Model file for the job. Use its own axes, mm. A direction names the side the tool comes from. Round coordinates to 2 decimals unless told otherwise and drop trailing zeros. Put each result on its own line as item: value. Start each with the question number.
Item 1: Pin check, flat tips, straight feed: pin 1 Ø8 at (x, y) = (124, 31.57) entering from -Z; pin 2 Ø7 at (x, y) = (124, 33.5) entering from -Z; pin 3 Ø6 at (x, y) = (136.5, 17) entering from -Z; pin 4 Ø4 at (y, z) = (27.5, 3.5) entering from -X. Stop position of each tip, or through.
Item 2: Mould opens along Y. For faces 1 (the face through (134.33, 18.47, 3.53)), 2 (the face through (146.229, 21, -4)), 3 (the face through (104.15, 5.837, -9.68)) say: pulls with the +Y half, pulls with the -Y half, needs draft (parallel to the pull), parting line crosses it, or undercut.
Item 3: Which spindle directions (+Z, -Z, +X, -X, +Y, -Y) get a long thin tool onto all of the face, cutting with end or side? Do faces 4 (the face through (128, 11, 1.27)), 5 (the face through (102.2, 21.2, -10.6)). Say none if no direction does.
Item 4: Probe probe 1 along Y at (x, z) = (116.5, -5.5); probe 2 along X at (y, z) = (17.5, -2); probe 3 along X at (y, z) = (19, -2.75). List the from-to ranges inside material, lowest first.
Item 5: Saw through at B-B on z = -2.75. State how many separate pieces and enclosed holes the cut face has, plus the area to 3 significant figures.
```python
from build123d import *

# Parameters (mm, degrees)
SKETCH1_W                   = 44.45
SKETCH1_H                   = 33.86758938
SKETCH1_W_2                 = 38.1
SKETCH1_H_2                 = 32.59758938
BOSS_EXTRUDE1_DEPTH         = 6.35
SKETCH2_W                   = 44.45
SKETCH2_H                   = 33.86758938
BOSS_EXTRUDE2_DEPTH         = 9.525
CUT_EXTRUDE1_DEPTH          = 151.402114191
SKETCH4_W                   = 3.175
SKETCH4_H                   = 33.86758938
BOSS_EXTRUDE3_DEPTH         = 4.7625
SHELL2_START                = 9.24120531
SHELL2_DEPTH                = 24.34258938
FILLET4_R                   = 4.7625
FILLET1_R                   = 4.7625
FILLET3_R                   = 6.35
FILLET2_R                   = 1.5875
F_10_CLEARANCE_HOLE1_D      = 5.6134
F_10_CLEARANCE_HOLE1_DEPTH  = 7.802129636
BOSS_EXTRUDE4_REACH         = 152.369
CUT_EXTRUDE2_START          = -4.7625
SKETCH9_R                   = 6.82625
CUT_EXTRUDE2_DEPTH          = 145.161286958
HOLE1_AT_2_COUNT            = 2
HOLE1_AT_2_PITCH            = 20.32
F_1_4_CLEARANCE_HOLE1_D     = 7.14248
F_1_4_CLEARANCE_HOLE1_DEPTH = 9.652
F_1_4_CLEARANCE_HOLE1_TIP   = 2.145817477


# Read off the part's stored shape, not the designer's step: Shell2
with BuildPart() as part:
    # Sketch1 → Boss-Extrude1 (new body)
    with BuildSketch(Plane.XY):
        with Locations((124.004465969, 21.4125)):
            Rectangle(SKETCH1_W, SKETCH1_H)
        with Locations((124.004465969, 21.4125)):
            Rectangle(SKETCH1_W_2, SKETCH1_H_2, mode=Mode.SUBTRACT)
    extrude(amount=-BOSS_EXTRUDE1_DEPTH)

    # Sketch2 → Boss-Extrude2 (add)
    with BuildSketch(Plane.XY):
        with Locations((124.004465969, 21.4125)):
            Rectangle(SKETCH2_W, SKETCH2_H)
    extrude(amount=BOSS_EXTRUDE2_DEPTH)

    # Sketch3 → Cut-Extrude1 (cut, through all)
    with BuildSketch(Plane.XZ.offset(-4.47870531)):
        Polygon((130.354465969, 9.525), (146.229465969, 5.27130657), (146.229465969, 9.525), align=None)
        Polygon((101.779465969, 9.525), (117.654465969, 9.525), (101.779465969, 5.27130657), align=None)
    extrude(amount=-CUT_EXTRUDE1_DEPTH, mode=Mode.SUBTRACT)

    # Sketch4 → Boss-Extrude3 (add)
    with BuildSketch(Plane(origin=(0, 0, -6.35), x_dir=(-1, 0, 0), z_dir=(0, 0, -1))):
        with Locations((-144.641965969, 21.4125)):
            Rectangle(SKETCH4_W, SKETCH4_H)
        with Locations((-103.366965969, 21.4125)):
            Rectangle(SKETCH4_W, SKETCH4_H)
    extrude(amount=BOSS_EXTRUDE3_DEPTH)

    # Shell2 outline → Shell2 (cut)
    with BuildSketch(Plane(origin=(0, 0, 0), x_dir=(1, 0, 0), z_dir=(0, 1, 0)).offset(SHELL2_START)):
        Polygon((141.466965969, 0), (106.541965969, 0), (106.541965969, -1.61691179), (118.281460989, -4.7625), (129.727470949, -4.7625), (141.466965969, -1.61691179), align=None)
    extrude(amount=SHELL2_DEPTH, mode=Mode.SUBTRACT)

    # Fillet4
    fillet4_edges = [part.edges().sort_by_distance(p)[0] for p in [
        (144.641965969, 38.34629469, -11.1125),
        (103.366965969, 38.34629469, -11.1125),
        (144.641965969, 4.47870531, -11.1125),
        (103.366965969, 4.47870531, -11.1125),
    ]]
    fillet(fillet4_edges, radius=FILLET4_R)

    # Fillet1
    fillet1_edges = [part.edges().sort_by_distance(p)[0] for p in [
        (146.229465969, 21.4125, 5.27130657),
        (101.779465969, 21.4125, 5.27130657),
    ]]
    fillet(fillet1_edges, radius=FILLET1_R)

    # Fillet3
    fillet3_edges = [part.edges().sort_by_distance(p)[0] for p in [
        (130.354465969, 21.4125, 9.525),
        (117.654465969, 21.4125, 9.525),
    ]]
    fillet(fillet3_edges, radius=FILLET3_R)

    # Fillet2
    fillet2_edges = [part.edges().sort_by_distance(p)[0] for p in [
        (146.229465969, 21.4125, -11.1125),
        (146.229465969, 4.47870531, -2.366544105),
        (146.229465969, 38.34629469, -2.366544105),
        (146.229465969, 5.873609265, -9.717596045),
        (146.229465969, 36.951390735, -9.717596045),
        (101.779465969, 38.34629469, -2.366544105),
        (101.779465969, 21.4125, -11.1125),
        (101.779465969, 4.47870531, -2.366544105),
        (101.779465969, 5.873609265, -9.717596045),
        (101.779465969, 36.951390735, -9.717596045),
        (111.07814933, 4.47870531, 7.762881267),
        (102.763620686, 4.47870531, 4.516138096),
        (145.245311252, 4.47870531, 4.516138096),
        (111.07814933, 38.34629469, 7.762881267),
        (102.763620686, 38.34629469, 4.516138096),
        (145.245311252, 38.34629469, 4.516138096),
        (124.004465969, 38.34629469, 9.525),
        (124.004465969, 4.47870531, 9.525),
        (136.930782609, 4.47870531, 7.762881267),
        (130.34731393, 4.47870531, 9.47067487),
        (117.661618008, 4.47870531, 9.47067487),
        (136.930782609, 38.34629469, 7.762881267),
        (130.34731393, 38.34629469, 9.47067487),
        (117.661618008, 38.34629469, 9.47067487),
    ]]
    fillet(fillet2_edges, radius=FILLET2_R)

    # #10 Clearance Hole1
    with Locations(Plane(origin=(5.500104786, 0, -20.526670507), x_dir=(0.96592582628907, 0, 0.2588190451025144), z_dir=(-0.2588190451025144, 0, 0.96592582628907))):
        with Locations((109.302434691, 21.4125)):
            f_10_clearance_hole1 = Hole(F_10_CLEARANCE_HOLE1_D / 2, depth=F_10_CLEARANCE_HOLE1_DEPTH)

    # Mirror1: #10 Clearance Hole1 across plane
    add(f_10_clearance_hole1.mirror(Plane(origin=(124.004465969, 0, 0), x_dir=(0, 0, 1), z_dir=(1, 0, 0))), mode=Mode.SUBTRACT)

    # Sketch8 → Boss-Extrude4 (add, up to next)
    with BuildSketch(Plane(origin=(0, 5.11370531, 0), x_dir=(1, 0, 0), z_dir=(0, 1, 0)), mode=Mode.PRIVATE) as boss_extrude4_sk1:
        Polygon((106.541965969, 0), (106.541965969, -1.61691179), (118.281460989, -4.7625), (129.727470949, -4.7625), (141.466965969, -1.61691179), (141.466965969, 0), (143.054465969, 0), (143.054465969, 6.35), (104.954465969, 6.35), (104.954465969, 0), align=None)
    boss_extrude4_tool1 = extrude(boss_extrude4_sk1.sketch, amount=BOSS_EXTRUDE4_REACH, mode=Mode.PRIVATE) - part.part
    add(boss_extrude4_tool1.solids().sort_by_distance((124.004466, 5.113705, -1.371306))[0])

    # Sketch9 → Cut-Extrude2 (cut, through all)
    with BuildSketch(Plane(origin=(5.500104786, 0, -20.526670507), x_dir=(0.96592582628907, 0, 0.2588190451025144), z_dir=(-0.2588190451025144, 0, 0.96592582628907)).offset(CUT_EXTRUDE2_START)):
        with Locations((109.302434691, 21.4125)):
            Circle(SKETCH9_R)
    cut_extrude2 = extrude(amount=-CUT_EXTRUDE2_DEPTH, mode=Mode.SUBTRACT)

    # Mirror2: Cut-Extrude2 across plane
    add(cut_extrude2.mirror(Plane(origin=(124.004465969, 0, 0), x_dir=(0, 0, 1), z_dir=(1, 0, 0))), mode=Mode.SUBTRACT)

    # Sketch12 → Hole1 (revolve, cut)
    with BuildSketch(Plane(origin=(124.004465969, 31.5725, -6.35), x_dir=(0, 1, 0), z_dir=(1, 0, 0))):
        Polygon((0, 0), (0, 7.62), (4.4323, 7.62), (4.6101, 0), align=None)
    hole1 = revolve(axis=Axis((124.004465969, 31.5725, 103.65), (0, 0, -1)), mode=Mode.SUBTRACT)

    # Hole1 at 2: Hole1 ×2
    with Locations(*[(0, -i * HOLE1_AT_2_PITCH, 0) for i in range(1, HOLE1_AT_2_COUNT)]):
        add(hole1, mode=Mode.SUBTRACT)

    # 1/4 Clearance Hole1
    with Locations(Plane(origin=(0, 0, -6.35), x_dir=(-1, 0, 0), z_dir=(0, 0, -1))):
        with Locations((-124.004465969, 11.2525), (-124.004465969, 31.5725)):
            Hole(F_1_4_CLEARANCE_HOLE1_D / 2, depth=F_1_4_CLEARANCE_HOLE1_DEPTH)
            with Locations((0, 0, -(F_1_4_CLEARANCE_HOLE1_DEPTH + F_1_4_CLEARANCE_HOLE1_TIP / 2))):  # 118° drill point
                Cone(0, F_1_4_CLEARANCE_HOLE1_D / 2, F_1_4_CLEARANCE_HOLE1_TIP, mode=Mode.SUBTRACT)


solid = part.part
```
Results found:
1. pin 1: stops at z = 1.27
1. pin 2: stops at z = -6.35
1. pin 3: stops at z = -6.35
1. pin 4: stops at x = 101.78
2. face 1: undercut
2. face 2: needs draft
2. face 3: pulls with the -Y half
3. face 4: -Z
3. face 5: -Z, -X, +Y, -Y
4. probe 1: y = 4.48 to 14.83, 28 to 38.35
4. probe 2: x = 101.78 to 107.9, 119.49 to 128.52, 140.11 to 146.23
4. probe 3: x = 101.78 to 107.28, 120.51 to 127.5, 140.72 to 146.23
5. separate pieces: 1
5. enclosed holes: 4
5. area: 1,070 mm²
